Part print with two shaded views. Sizes in mm from the minimum x, y, z corner. Round coordinates to 2 decimals unless told otherwise and drop trailing zeros. Loops run counter-clockwise (first coordinate to the right, second up) from the corner with the lowest first, then second, coordinate; pieces in that order, holes last. Notation, with made-up numbers: (56, 55) -> (98, 55) arc R14 cw to (98, 71) -> close; hole circle Ø9 at (19, 36.5). An arc over 180 degrees is marked (long way). Use a Markdown table: item, result. Add a question column.
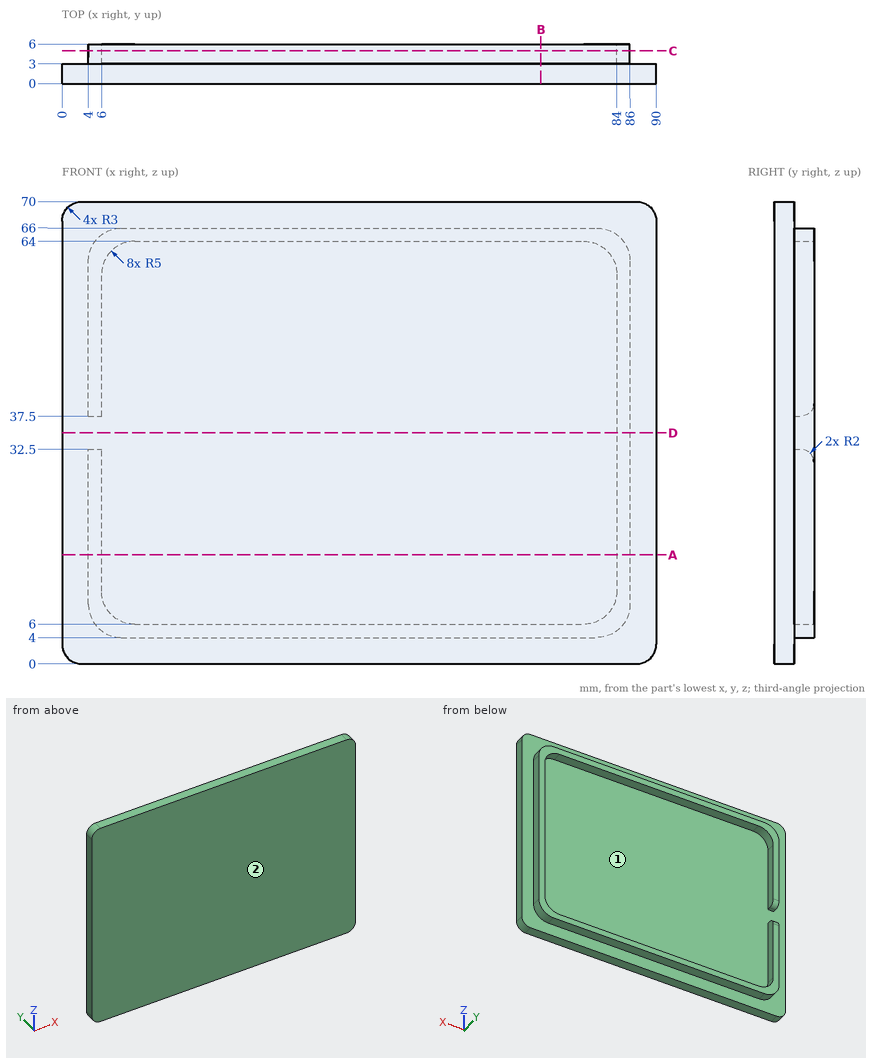
1) Pull direction Z, two halves, no side cores. Call the marked faces 1 and 2: +Z half, -Z half, draft (parallel to the pull), parting line (faces both ways), or undercut.
2) Cut at D-D on z = 35. Write the cut outline in (x, y).
3) Cut at C-C on y = 4.95. Write the cut outline in (x, z).
4) Wall check: probe 1 along X at (y, z) = (3.35, 41); probe 2 along Z at (x, y) = (46, 4.35); probe 3 along Y at (x, z) = (48.5, 58). Give the ranges that are in metal, low to high. Write a range as from..to.
5) Pin check, flat tips, straight feed: pin 1 Ø1.5 at (y, z) = (4.5, 25) entering from -X; pin 2 Ø0.9 at (y, z) = (4, 46) entering from +X; pin 3 Ø0.9 at (x, y) = (42, 4) entering from +Z. Stop position of each tip, or through.
6) Cut at A-A on z = 16.5. Write the cut outline in (x, y), and give its area (3 significant figures).
7) Cut at B-B on x = 72.5. Write the cut outline in (y, z).
Established:
| question | item | result |
|---|---|---|
| 1 | face 1 | undercut |
| 1 | face 2 | draft |
| 2 | outline | (0, 0) -> (90, 0) -> (90, 3) -> (86, 3) -> (86, 6) -> (84, 6) -> (84, 3) -> (0, 3) -> close |
| 3 | outline | (4, 9) arc R5 ccw to (9, 4) -> (81, 4) arc R5 ccw to (86, 9) -> (86, 61) arc R5 ccw to (81, 66) -> (9, 66) arc R5 ccw to (4, 61) -> (4, 37.74) -> (6, 37.74) -> (6, 59) arc R5 cw to (11, 64) -> (79, 64) arc R5 cw to (84, 59) -> (84, 11) arc R5 cw to (79, 6) -> (11, 6) arc R5 cw to (6, 11) -> (6, 32.26) -> (4, 32.26) -> close |
| 4 | probe 1 | x = 4..6, 84..86 |
| 4 | probe 2 | z = 4..6, 64..66 |
| 4 | probe 3 | y = 0..3 |
| 5 | pin 1 | stops at x = 4 |
| 5 | pin 2 | stops at x = 86 |
| 5 | pin 3 | stops at z = 66 |
| 6 | outline | (0, 0) -> (90, 0) -> (90, 3) -> (86, 3) -> (86, 6) -> (84, 6) -> (84, 3) -> (6, 3) -> (6, 6) -> (4, 6) -> (4, 3) -> (0, 3) -> close |
| 6 | area | 282 mm^2 |
| 7 | outline | (0, 0) -> (3, 0) -> (3, 4) -> (6, 4) -> (6, 6) -> (3, 6) -> (3, 64) -> (6, 64) -> (6, 66) -> (3, 66) -> (3, 70) -> (0, 70) -> close |
